from build123d import *

# Parameters (mm, degrees)
SKETCH1_W                = 53.621579066
SKETCH1_H                = 6.35
BOSS_EXTRUDE2_DEPTH      = 63.5
CUT_EXTRUDE2_DEPTH       = 93.248761228
CUT_EXTRUDE2_DEPTH_BACK  = 0.762
SKETCH3_R                = 1.5875
SKETCH5_R                = 10.16
SKETCH5_R_2              = 1.27
BOSS_EXTRUDE3_DEPTH      = 3.175
BOSS_EXTRUDE4_START      = 3.175
SKETCH6_R                = 10.16
SKETCH6_R_2              = 1.27
BOSS_EXTRUDE4_DEPTH      = 3.175
SKETCH11_W               = 7.62
SKETCH11_H               = 22.225
SKETCH11_H_2             = 28.067
SKETCH11_W_2             = 10.16
SKETCH11_H_3             = 3.175
CUT_EXTRUDE10_DEPTH      = 96.056489111
CUT_EXTRUDE11_DEPTH      = 81.036983958
CUT_EXTRUDE11_DEPTH_BACK = 81.036983958
SKETCH12_W               = 4.7625
SKETCH12_H               = 15.24
CUT_EXTRUDE12_DEPTH      = 96.056489111


with BuildPart() as part:
    # Sketch1 → Boss-Extrude2 (new body)
    with BuildSketch(Plane.XY):
        with Locations((-39.51078952, 5.715)):
            Rectangle(SKETCH1_W, SKETCH1_H)
    extrude(amount=BOSS_EXTRUDE2_DEPTH)

    # Sketch3 → Cut-Extrude2 (cut, two sides: drawn at the far end of the back side and taken through both)
    with BuildSketch(Plane(origin=(0, 0, 63.5), x_dir=(-1, 0, 0), z_dir=(0, 0, -1)).offset(-CUT_EXTRUDE2_DEPTH_BACK)):
        with Locations((17.3355, 5.715)):
            Circle(SKETCH3_R)
    extrude(amount=CUT_EXTRUDE2_DEPTH + CUT_EXTRUDE2_DEPTH_BACK, mode=Mode.SUBTRACT)

    # Sketch5 → Boss-Extrude3 (add)
    with BuildSketch(Plane.XY.offset(63.5)):
        with Locations(Location((-30.1625, 12.573, 0), (0, 0, 201.253809185))):
            Circle(SKETCH5_R)
        with Locations((-30.1625, 12.573)):
            Circle(SKETCH5_R_2, mode=Mode.SUBTRACT)
    extrude(amount=BOSS_EXTRUDE3_DEPTH)

    # Sketch6 → Boss-Extrude4 (add)
    with BuildSketch(Plane(origin=(0, 0, 0), x_dir=(-1, 0, 0), z_dir=(0, 0, -1)).offset(BOSS_EXTRUDE4_START)):
        with Locations(Location((30.1625, 12.573, 0), (0, 0, 338.746190815))):
            Circle(SKETCH6_R)
        with Locations(Location((30.1625, 12.573, 0), (0, 0, 180))):
            Circle(SKETCH6_R_2, mode=Mode.SUBTRACT)
    extrude(amount=-BOSS_EXTRUDE4_DEPTH)

    # Sketch11 → Cut-Extrude10 (cut, through all)
    with BuildSketch(Plane(origin=(0, 8.89, 0), x_dir=(1, 0, 0), z_dir=(0, 1, 0))):
        with Locations((-16.509999987, -11.1125)):
            Rectangle(SKETCH11_W, SKETCH11_H)
        with Locations((-16.509999987, -49.4665)):
            Rectangle(SKETCH11_W, SKETCH11_H_2)
        with Locations((-17.779999987, -28.829)):
            Rectangle(SKETCH11_W_2, SKETCH11_H_3)
    extrude(amount=-CUT_EXTRUDE10_DEPTH, mode=Mode.SUBTRACT)

    # Sketch10 → Cut-Extrude11 (cut, two sides: drawn at the far end of the back side and taken through both)
    with BuildSketch(Plane.XY.offset(35.433).offset(-CUT_EXTRUDE11_DEPTH_BACK)):
        with BuildLine():
            Line((-12.699999987, 8.89), (-15.068097359, 8.89))
            ThreePointArc((-15.068097359, 8.89), (-13.401759428, 7.757904548), (-12.699999987, 5.86955715))
            Line((-12.699999987, 5.86955715), (-12.699999987, 8.89))
        make_face()
        with BuildLine():
            Line((-12.699999987, 2.54), (-12.699999987, 5.56044285))
            ThreePointArc((-12.699999987, 5.56044285), (-13.401759428, 3.672095452), (-15.068097359, 2.54))
            Line((-15.068097359, 2.54), (-12.699999987, 2.54))
        make_face()
    extrude(amount=CUT_EXTRUDE11_DEPTH + CUT_EXTRUDE11_DEPTH_BACK, mode=Mode.SUBTRACT)

    # Sketch12 → Cut-Extrude12 (cut, through all)
    with BuildSketch(Plane(origin=(0, 8.89, 0), x_dir=(1, 0, 0), z_dir=(0, 1, 0))):
        with Locations((-22.701249987, -7.62)):
            Rectangle(SKETCH12_W, SKETCH12_H)
        with Locations((-22.701249987, -55.88)):
            Rectangle(SKETCH12_W, SKETCH12_H)
    extrude(amount=-CUT_EXTRUDE12_DEPTH, mode=Mode.SUBTRACT)


solid = part.part
For this review, take the finished solid that the model builds, in its own axes (mm). A direction names the side the tool comes from. Give positions to 0.01 mm unless a question says otherwise; leave off trailing zeros. Loops run counter-clockwise (first coordinate to the right, second up) from the corner with the lowest first, then second, coordinate; pieces in that order, holes last. Notation, with made-up numbers: (66.25, 70.25) -> (89.25, 70.25) arc R28 cw to (89.25, 97.25) -> close; hole circle Ø5 at (38, 84). An arc over 180 degrees is marked (long way). One line per question, with ' | ' between items.
1) Insertion check: pin 1 Ø12 at (x, y) = (-50, 5.5) entering from -Z; pin 2 Ø1.9 at (x, y) = (-52.5, 6) entering from +Z; pin 3 Ø1.9 at (y, z) = (5, 19.5) entering from +X; pin 4 Ø2.5 at (x, y) = (-17.34, 5.72) entering from -Z. Each pin has a flat end and moves straight along its axis. Give the tip position at first contact, or say it passes through.
Resolved:
pin 1: stops at z = 0 | pin 2: stops at z = 63.5 | pin 3: stops at x = -20.32 | pin 4: passes through
2) For faces 1 (the flat face through (-47, 2.54, 31)), 2 (the flat face through (-23, 6, 15.24)), 3 (the cylindrical face through (-40.32, 12.8, 65.07)), list the 3-axis set-ups (+Z, -Z, +X, -X, +Y, -Y) from which the entire face can be reached by the end or side of a thin tool; tool diameter is ignored.
Resolved:
face 1: +X, -X, -Y | face 2: +X, +Y, -Y | face 3: +Z
3) We need section C-C (z = 42.5). Write out the cut boundary in (x, y).
Resolved:
outline: (-66.32, 2.54) -> (-20.32, 2.54) -> (-20.32, 8.89) -> (-66.32, 8.89) -> close
4) The part is to be moulded in two halves that separate along Z. For faces 4 (the cylindrical face through (-15.75, 5.78, 32.96)), 5 (the flat face through (-29, 11, -3.175)), 6 (the flat face through (-19, 5, 30.416)), say which applies: +Z half, -Z half, draft (parallel to the pull), parting line (faces both ways), or undercut.
Resolved:
face 4: draft | face 5: -Z half | face 6: undercut
5) We need section B-B (y = 18.75). Write out the cut boundary in (x, z) (3 decimals), plus the area to 3 significant figures.
Resolved:
outline: (-38.229, -3.175) -> (-22.096, -3.175) -> (-22.096, 0) -> (-38.229, 0) -> close; (-38.229, 63.5) -> (-22.096, 63.5) -> (-22.096, 66.675) -> (-38.229, 66.675) -> close | area: 102 mm2
6) We need section A-A (x = -16.5). Write out the cut boundary in (y, z) (1 decimal), plus the area to 3 significant figures.
Resolved:
outline: (2.5, 22.2) -> (4.4, 22.2) -> (4.4, 27.2) -> (2.5, 27.2) -> close; (2.5, 30.4) -> (4.4, 30.4) -> (4.4, 35.4) -> (2.5, 35.4) -> close; (7.1, 22.2) -> (8.9, 22.2) -> (8.9, 27.2) -> (7.1, 27.2) -> close; (7.1, 30.4) -> (8.9, 30.4) -> (8.9, 35.4) -> (7.1, 35.4) -> close | area: 36.6 mm2
7) We need section D-D (x = -26.5). Write out the cut boundary in (y, z) (3 decimals), plus the area to 3 significant figures.
Resolved:
outline: (2.54, 0) -> (3.096, 0) -> (3.096, -3.175) -> (22.05, -3.175) -> (22.05, 0) -> (8.89, 0) -> (8.89, 63.5) -> (22.05, 63.5) -> (22.05, 66.675) -> (3.096, 66.675) -> (3.096, 63.5) -> (2.54, 63.5) -> close | area: 524 mm2
8) To check wall thickness, follow probe 1 along Z at (x, y) = (-20, 7.5) (1 decimal); probe 2 along Y at (x, z) = (-36.5, 37); probe 3 along Z at (x, y) = (-35.5, 18) (3 decimals). State the ranges of each line that lie inside material, in increasing order.
Resolved:
probe 1: z = 22.2 to 27.2, 30.4 to 35.4 | probe 2: y = 2.54 to 8.89 | probe 3: z = -3.175 to 0, 63.5 to 66.675
